Source: CAD feature listing. Evaluate the final solid. Frame: model axes, mm. Round coordinates to 2 decimals unless told otherwise and drop trailing zeros. Loops run counter-clockwise (first coordinate to the right, second up) from the corner with the lowest first, then second, coordinate; pieces in that order, holes last.
Item 1: Ray query, L1, parallel to Y at x = -62.5, z = 5.25; L2, parallel to Y at x = -44, z = 7.5; L3, parallel to Y at x = 7.5, z = 4.5. Return the intervals inside material, ascending.
Item 2: Section query C-C on x = 0. Return loops of the section in (y, z), then the cut area to 3 significant figures.
Item 3: Section query D-D on y = -7.5. Return loops of the section in (x, z), then the cut area to 4 significant figures.
Item 4: Section query A-A on y = 12.5. Return loops of the section in (x, z), then the cut area to 3 significant figures.
Item 5: Section query B-B on z = 13.25. Give the number of separate pieces and of enclosed holes in the cut face, then the cut area to 3 significant figures.
Item 6: First-contact query: P1, Ø5.5, axis at x = 8.5, y = 11.5, coming from the +Z side; P2, Ø12, axis at x = -8, y = 11, coming from the +Z side. Flat tips, straight axial feed; report the tip coordinate or a pass-through.
```python
from build123d import *

# Parameters (mm, degrees)
SKETCH_W        = 148
SKETCH_H        = 95
PAD_DEPTH       = 18
SKETCH001_R     = 3.3
SKETCH001_R_2   = 2.75
SKETCH001_R_3   = 2.1
POCKET_DEPTH    = 18.001
SKETCH002_R     = 5.5
POCKET001_DEPTH = 6.8
FILLET_R        = 6
SKETCH003_R     = 2.75
POCKET002_DEPTH = 18.001


with BuildPart() as part:
    # Sketch → Pad (new body)
    with BuildSketch(Plane.XY):
        Rectangle(SKETCH_W, SKETCH_H)
    extrude(amount=PAD_DEPTH)

    # Sketch001 (on Face6 of Pad) → Pocket (cut, through all)
    with BuildSketch(Plane.XY.offset(18)):
        with Locations((-62.5, 12.5)):
            Circle(SKETCH001_R)
        with Locations((-62.5, -27.5)):
            Circle(SKETCH001_R)
        with Locations((-9.5, 12.5)):
            Circle(SKETCH001_R)
        with Locations((-9.5, -27.5)):
            Circle(SKETCH001_R)
        with Locations((0, -7.5)):
            Circle(SKETCH001_R_2)
        with Locations((0, 23.5)):
            Circle(SKETCH001_R_2)
        with Locations((-68, 41.5)):
            Circle(SKETCH001_R_3)
        with Locations((-44, 41.5)):
            Circle(SKETCH001_R_3)
        with Locations((-17.5, 41.5)):
            Circle(SKETCH001_R_2)
        with Locations((9.5, -27.5)):
            Circle(SKETCH001_R)
        with Locations((9.5, 12.5)):
            Circle(SKETCH001_R)
        with Locations((17.5, 41.5)):
            Circle(SKETCH001_R_2)
        with Locations((44, 41.5)):
            Circle(SKETCH001_R_3)
        with Locations((68, 41.5)):
            Circle(SKETCH001_R_3)
        with Locations((62.5, 12.5)):
            Circle(SKETCH001_R)
        with Locations((62.5, -27.5)):
            Circle(SKETCH001_R)
    extrude(amount=-POCKET_DEPTH, mode=Mode.SUBTRACT)

    # Sketch002 → Pocket001 (cut)
    with BuildSketch(Plane.XY.offset(18)):
        with Locations((-9.5, 12.5)):
            Circle(SKETCH002_R)
        with Locations((9.5, 12.5)):
            Circle(SKETCH002_R)
        with Locations((-9.5, -27.5)):
            Circle(SKETCH002_R)
        with Locations((9.5, -27.5)):
            Circle(SKETCH002_R)
        with Locations((0, 23.5)):
            Circle(SKETCH002_R)
    extrude(amount=-POCKET001_DEPTH, mode=Mode.SUBTRACT)

    # Fillet
    fillet_edges = [part.edges().sort_by_distance(p)[0] for p in [
        (-74, 47.5, 9),
        (74, 47.5, 9),
    ]]
    fillet(fillet_edges, radius=FILLET_R)

    # Sketch003 (on Face5 of Fillet) → Pocket002 (cut, through all)
    with BuildSketch(Plane.XY.offset(18)):
        with Locations((0, -7.5)):
            Circle(SKETCH003_R)
        with Locations((0, 23.5)):
            Circle(SKETCH003_R)
    extrude(amount=-POCKET002_DEPTH, mode=Mode.SUBTRACT)


solid = part.part
```
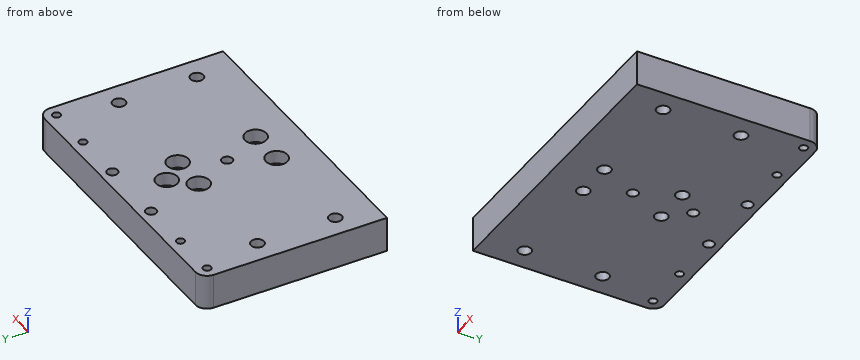
Data:
1. L1: y = -47.5 to -30.8, -24.2 to 9.2, 15.8 to 47.5
1. L2: y = -47.5 to 39.4, 43.6 to 47.5
1. L3: y = -47.5 to -30.12, -24.88 to 9.88, 15.12 to 47.5
2. outline: (-47.5, 0) - (-10.25, 0) - (-10.25, 18) - (-47.5, 18) - close; (-4.75, 0) - (20.75, 0) - (20.75, 11.2) - (18, 11.2) - (18, 18) - (-4.75, 18) - close; (26.25, 0) - (47.5, 0) - (47.5, 18) - (29, 18) - (29, 11.2) - (26.25, 11.2) - close
2. area: 1,470 mm2
3. outline: (-74, 0) - (-2.75, 0) - (-2.75, 18) - (-74, 18) - close; (2.75, 0) - (74, 0) - (74, 18) - (2.75, 18) - close
3. area: 2,565 mm2
4. outline: (-74, 0) - (-65.8, 0) - (-65.8, 18) - (-74, 18) - close; (-59.2, 0) - (-12.8, 0) - (-12.8, 11.2) - (-15, 11.2) - (-15, 18) - (-59.2, 18) - close; (-6.2, 0) - (6.2, 0) - (6.2, 11.2) - (4, 11.2) - (4, 18) - (-4, 18) - (-4, 11.2) - (-6.2, 11.2) - close; (12.8, 0) - (59.2, 0) - (59.2, 18) - (15, 18) - (15, 11.2) - (12.8, 11.2) - close; (65.8, 0) - (74, 0) - (74, 18) - (65.8, 18) - close
4. area: 2,130 mm2
5. separate pieces: 1
5. enclosed holes: 16
5. area: 13,300 mm2
6. P1: stops at z = 11.2
6. P2: stops at z = 18
